```python
from build123d import *

# Parameters (mm, degrees)
SKETCH1_W           = 42
SKETCH1_H           = 32
SKETCH1_R           = 1.6
BOSS_EXTRUDE1_DEPTH = 2
FILLET1_R           = 1


with BuildPart() as part:
    # Sketch1 → Boss-Extrude1 (new body)
    with BuildSketch(Plane(origin=(0, 0, 0), x_dir=(1, 0, 0), z_dir=(0, 1, 0))):
        Rectangle(SKETCH1_W, SKETCH1_H)
        with Locations(Location((-18.5, 0, 0), (0, 0, 270))):
            Circle(SKETCH1_R, mode=Mode.SUBTRACT)
        with Locations(Location((18.5, 0, 0), (0, 0, 90))):
            Circle(SKETCH1_R, mode=Mode.SUBTRACT)
    extrude(amount=BOSS_EXTRUDE1_DEPTH)

    # Fillet1
    # the kernel refuses this fillet: 1 mm, written as the material it takes off along each edge
    with BuildSketch(Plane(origin=(-20, 1, -15), x_dir=(-1, 0, 0), z_dir=(0, 0, -1))) as fillet1_piece_1_section:
        Polygon((0, 0), (FILLET1_R, 0), (FILLET1_R, FILLET1_R), (0, FILLET1_R), align=None)
    fillet1_piece_1 = extrude(amount=FILLET1_R, mode=Mode.PRIVATE)
    fillet1_piece_1 = fillet1_piece_1 - Plane(origin=(-20, 1, -15), x_dir=(0.7071067811865475, -0.7071067811865475, 0), z_dir=(0, 0, -1)) * Sphere(FILLET1_R, mode=Mode.PRIVATE)
    add(fillet1_piece_1, mode=Mode.SUBTRACT)
    with BuildSketch(Plane(origin=(-20, 1, 15), x_dir=(-1, 0, 0), z_dir=(0, 0, 1))) as fillet1_piece_2_section:
        Polygon((0, 0), (FILLET1_R, 0), (FILLET1_R, -FILLET1_R), (0, -FILLET1_R), align=None)
    fillet1_piece_2 = extrude(amount=FILLET1_R, mode=Mode.PRIVATE)
    fillet1_piece_2 = fillet1_piece_2 - Plane(origin=(-20, 1, 15), x_dir=(0.7071067811865475, -0.7071067811865475, 0), z_dir=(0, 0, 1)) * Sphere(FILLET1_R, mode=Mode.PRIVATE)
    add(fillet1_piece_2, mode=Mode.SUBTRACT)
    with BuildSketch(Plane(origin=(20, 1, 15), x_dir=(1, 0, 0), z_dir=(0, 0, 1))) as fillet1_piece_3_section:
        Polygon((0, 0), (FILLET1_R, 0), (FILLET1_R, FILLET1_R), (0, FILLET1_R), align=None)
    fillet1_piece_3 = extrude(amount=FILLET1_R, mode=Mode.PRIVATE)
    fillet1_piece_3 = fillet1_piece_3 - Plane(origin=(20, 1, 15), x_dir=(-0.7071067811865475, -0.7071067811865475, 0), z_dir=(0, 0, 1)) * Sphere(FILLET1_R, mode=Mode.PRIVATE)
    add(fillet1_piece_3, mode=Mode.SUBTRACT)
    with BuildSketch(Plane(origin=(20, 1, -15), x_dir=(0, 0, -1), z_dir=(1, 0, 0))) as fillet1_piece_4_section:
        Polygon((0, 0), (FILLET1_R, 0), (FILLET1_R, FILLET1_R), (0, FILLET1_R), align=None)
    fillet1_piece_4 = extrude(amount=FILLET1_R, mode=Mode.PRIVATE)
    fillet1_piece_4 = fillet1_piece_4 - Plane(origin=(20, 1, -15), x_dir=(0, -0.7071067811865475, 0.7071067811865475), z_dir=(1, 0, 0)) * Sphere(FILLET1_R, mode=Mode.PRIVATE)
    add(fillet1_piece_4, mode=Mode.SUBTRACT)
    with BuildSketch(Plane(origin=(-21, 2, -15), x_dir=(0, -1, 0), z_dir=(0, 0, 1)), Plane(origin=(21, 2, 15), x_dir=(0, -1, 0), z_dir=(0, 0, -1))) as fillet1_piece_5:
        with BuildLine():
            CenterArc((FILLET1_R, FILLET1_R), FILLET1_R, 180, 90)
            Line((0, FILLET1_R), (0, 0))
            Line((0, 0), (FILLET1_R, 0))
        make_face()
    extrude(amount=30, mode=Mode.SUBTRACT)
    with BuildSketch(Plane(origin=(-20, 2, 16), x_dir=(0, -1, 0), z_dir=(1, 0, 0)), Plane(origin=(20, 2, -16), x_dir=(0, -1, 0), z_dir=(-1, 0, 0))) as fillet1_piece_6:
        with BuildLine():
            CenterArc((FILLET1_R, FILLET1_R), FILLET1_R, 180, 90)
            Line((0, FILLET1_R), (0, 0))
            Line((0, 0), (FILLET1_R, 0))
        make_face()
    extrude(amount=40, mode=Mode.SUBTRACT)
    with BuildSketch(Plane(origin=(21, -2.5, 16), x_dir=(-1, 0, 0), z_dir=(0, 1, 0)), Plane(origin=(-21, -2.5, -16), x_dir=(1, 0, 0), z_dir=(0, 1, 0)), Plane(origin=(21, -2.5, -16), x_dir=(0, 0, 1), z_dir=(0, 1, 0))) as fillet1_piece_7:
        with BuildLine():
            CenterArc((FILLET1_R, -FILLET1_R), FILLET1_R, 90, 90)
            Line((0, -FILLET1_R), (0, 0))
            Line((0, 0), (FILLET1_R, 0))
        make_face()
    extrude(amount=3.5, mode=Mode.SUBTRACT)
    with BuildSketch(Plane(origin=(-21, -2.5, 16), x_dir=(1, 0, 0), z_dir=(0, 1, 0))) as fillet1_piece_8:
        with BuildLine():
            CenterArc((FILLET1_R, FILLET1_R), FILLET1_R, 180, 90)
            Line((0, FILLET1_R), (0, 0))
            Line((0, 0), (FILLET1_R, 0))
        make_face()
    extrude(amount=3.5, mode=Mode.SUBTRACT)


solid = part.part
```
Work out the finished part from the listing and answer in its coordinate system (mm). Give positions to 0.01 mm unless a question says otherwise; leave off trailing zeros. Order: outer loops, then holes, each group sorted by start corner. A loop starts at its lowest first (then second) coordinate and runs counter-clockwise, first axis right, second up. Notation, with made-up numbers: (56, 37) - (100, 37) arc R32 cw to (100, 74) - close; hole circle Ø3 at (-37, -23). An arc over 180 degrees is marked (long way). One line per item, written item: value. Start each with the question number.
1. Section B-B, the plane z = 0 is taken. Write down the section's boundary in (x, y).
2. Section A-A, the plane x = -18.5 is taken. Write down the section's boundary in (y, z), then the cut area to 3 significant figures.
3. Section C-C, the plane y = 1.4 is taken. Write down the section's boundary in (x, z).
4. For a pull along Z with two mould halves and no side action, classify faces 1 (the face through (-0.3, 0.5, 16)), 2 (the face through (-21, 0.5, 0.2)), 3 (the face through (-16.914, 0.986, -0.208)) as released by +Z, released by -Z, zero draft, split by the parting line, or undercut.
5. Consider line 1 (X direction, y = 0.85, z = 0); line 2 (Z direction, x = 18.5, y = 0.75); line 3 (X direction, y = 0.3, z = 1). Determine where each line is inside the solid, lowest interval first.
Filled sheet:
1. outline: (-21, 0) - (-20.1, 0) - (-20.1, 1.99) arc R1 ccw to (-21, 1) - close; (-16.9, 0) - (16.9, 0) - (16.9, 2) - (-16.9, 2) - close; (20.1, 0) - (21, 0) - (21, 1) arc R1 ccw to (20.1, 1.99) - close
2. outline: (0, -16) - (1, -16) arc R1 ccw to (2, -15) - (2, -1.6) - (0, -1.6) - close; (0, 1.6) - (2, 1.6) - (2, 15) arc R1 ccw to (1, 16) - (0, 16) - close
2. area: 57.2 mm²
3. outline: (-20.92, -15) arc R0.92 ccw to (-20, -15.92) - (20, -15.92) arc R0.92 ccw to (20.92, -15) - (20.92, 15) arc R0.92 ccw to (20, 15.92) - (-20, 15.92) arc R0.92 ccw to (-20.92, 15) - close; hole circle Ø3.2 at (-18.5, 0); hole circle Ø3.2 at (18.5, 0)
4. face 1: released by +Z
4. face 2: zero draft
4. face 3: undercut
5. line 1: -21 to -20.1, -16.9 to 16.9, 20.1 to 21
5. line 2: -16 to -1.6, 1.6 to 16
5. line 3: -21 to -19.75, -17.25 to 17.25, 19.75 to 21
